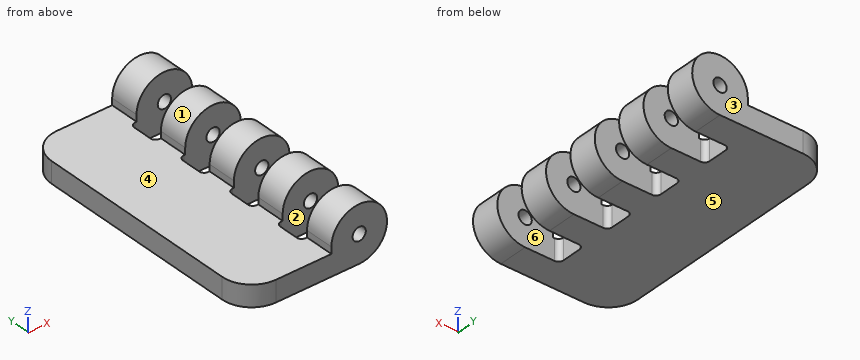
```python
from build123d import *

# Parameters (mm, degrees)
BOSS_EXTRUDE1_START = 31.75
SKETCH3_R           = 1.5875
BOSS_EXTRUDE1_DEPTH = 63.5
FILLET1_R           = 7.055555556
SKETCH5_W           = 16.383
SKETCH5_H           = 7.055555556
CUT_EXTRUDE1_DEPTH  = 43.200038063
LPATTERN1_COUNT     = 5
LPATTERN1_PITCH     = 14.111111111
FILLET2_R           = 1.175925926
SKETCH6_W           = 16.383
SKETCH6_H           = 7.055555555
CUT_EXTRUDE2_DEPTH  = 43.200038063
LPATTERN2_COUNT     = 4
LPATTERN2_PITCH     = 14.111111111
FILLET3_R           = 1.175925926
FILLET4_R           = 0.391975309
BOSS_EXTRUDE3_START = 31.75
SKETCH7_R           = 1.5875
BOSS_EXTRUDE3_DEPTH = 63.5


with BuildPart() as part:
    # Sketch3 → Boss-Extrude1 (new body)
    with BuildSketch(Plane(origin=(0, 0, 0), x_dir=(1, 0, 0), z_dir=(0, 1, 0)).offset(BOSS_EXTRUDE1_START)):
        with BuildLine():
            Line((26.9875, 6.6675), (26.9875, 1.5875))
            Line((26.9875, 1.5875), (6.6675, 1.5875))
            Line((6.6675, 1.5875), (6.6675, 0))
            ThreePointArc((6.6675, 0), (-4.714634464, -4.714634464), (0, 6.6675))
            Line((0, 6.6675), (26.9875, 6.6675))
        make_face()
        with Locations(Location((0, 0, 0), (0, 0, 270))):
            Circle(SKETCH3_R, mode=Mode.SUBTRACT)
    extrude(amount=-BOSS_EXTRUDE1_DEPTH)

    # Fillet1
    fillet1_edges = [part.edges().sort_by_distance(p)[0] for p in [
        (26.9875, -31.75, -4.1275),
        (26.9875, 31.75, -4.1275),
    ]]
    fillet(fillet1_edges, radius=FILLET1_R)


with BuildPart() as body_2:
    # Mirror1: mirrored copy
    add(part.part.mirror(Plane(origin=(0, 0, 0), x_dir=(0, 0, 1), z_dir=(1, 0, 0))))

    # Sketch6 → Cut-Extrude2 (cut, symmetric)
    with BuildSketch(Plane.XY):
        with Locations((0, 21.166666666)):
            Rectangle(SKETCH6_W, SKETCH6_H)
    cut_extrude2 = extrude(amount=CUT_EXTRUDE2_DEPTH, both=True, mode=Mode.SUBTRACT)

    # LPattern2: Cut-Extrude2 ×4
    with Locations(*[(0, -i * LPATTERN2_PITCH, 0) for i in range(1, LPATTERN2_COUNT)]):
        add(cut_extrude2, mode=Mode.SUBTRACT)

    # Fillet3
    fillet3_edges = [body_2.edges().sort_by_distance(p)[0] for p in [
        (-8.1915, 10.583333333, -4.1275),
        (-8.1915, 3.527777778, -4.1275),
        (-8.1915, -3.527777778, -4.1275),
        (-8.1915, -10.583333333, -4.1275),
        (-8.1915, -17.638888889, -4.1275),
        (-8.1915, -24.694444444, -4.1275),
        (-8.1915, 24.694444444, -4.1275),
        (-8.1915, 17.638888889, -4.1275),
    ]]
    fillet(fillet3_edges, radius=FILLET3_R)


with BuildPart() as part_1:
    add(part.part)

    # Sketch5 → Cut-Extrude1 (cut, symmetric)
    with BuildSketch(Plane.XY):
        with Locations((0, 28.222222222)):
            Rectangle(SKETCH5_W, SKETCH5_H)
    cut_extrude1 = extrude(amount=CUT_EXTRUDE1_DEPTH, both=True, mode=Mode.SUBTRACT)

    # LPattern1: Cut-Extrude1 ×5
    with Locations(*[(0, -i * LPATTERN1_PITCH, 0) for i in range(1, LPATTERN1_COUNT)]):
        add(cut_extrude1, mode=Mode.SUBTRACT)

    # Fillet2
    fillet2_edges = [part_1.edges().sort_by_distance(p)[0] for p in [
        (8.1915, -3.527777778, -4.1275),
        (8.1915, 3.527777778, -4.1275),
        (8.1915, -17.638888889, -4.1275),
        (8.1915, -10.583333333, -4.1275),
        (8.1915, -24.694444444, -4.1275),
        (8.1915, 24.694444444, -4.1275),
        (8.1915, 10.583333333, -4.1275),
        (8.1915, 17.638888889, -4.1275),
    ]]
    fillet(fillet2_edges, radius=FILLET2_R)

    # Fillet4
    fillet4_edges = [part_1.edges().sort_by_distance(p)[0] for p in [
        (8.1915, -31.75, -4.1275),
        (8.1915, 31.75, -4.1275),
    ]]
    fillet(fillet4_edges, radius=FILLET4_R)


with BuildPart() as body_3:
    # Sketch7 → Boss-Extrude3 (new body)
    with BuildSketch(Plane(origin=(0, 0, 0), x_dir=(1, 0, 0), z_dir=(0, 1, 0)).offset(BOSS_EXTRUDE3_START)):
        with Locations(Location((0, 0, 0), (0, 0, 270))):
            Circle(SKETCH7_R)
    extrude(amount=-BOSS_EXTRUDE3_DEPTH)


solid = body_2.part
```
Source: CAD feature listing. Evaluate the final solid. Frame: model axes, mm. Face numbers are marked on the shaded views. A direction names the side the tool comes from. Give positions to 0.01 mm unless a question says otherwise; leave off trailing zeros. Order: outer loops, then holes, each group sorted by start corner. A loop starts at its lowest first (then second) coordinate and runs counter-clockwise, first axis right, second up.
(1) Section query C-C (x = 3). Return the cut outline in (y, z).
(2) Access query for the marked faces 4, 5 and 6. Directions: +Z, -Z, +X, -X, +Y, -Y. A direction counts if a zero-diameter tool reaches every point of the face in a straight line with its end or side. Return the directions, or none.
(3) Section query D-D (y = 7.5). Return the cut outline in (x, z), plus the area to 3 significant figures.
(4) Pull-direction query (Y, two-part tool) for the marked faces 1, 2 and 3; classes: +Y half, -Y half, draft (parallel to the pull), parting line (faces both ways), or undercut.
(5) Section query A-A (z = 5.5). Return the cut outline in (x, y), plus the area to 3 significant figures.
(6) Section query B-B (y = 16). Return the cut outline in (x, z) (1 decimal).
(7) Material intervals for line 1 along Y through (x, z) = (1, 2.5); line 2 along X through (y, z) = (-1.75, 0); line 3 along Y through (x, z) = (-8, -2.75), sorted ascending.
(8) Contact query for flat-ended pins moving along their axis: P1, Ø1, axis at y = -21.5, z = -3.5, coming from the +X side; P2, Ø0.8, axis at y = -27, z = -0.5, coming from the -X side; P3, Ø2, axis at y = 1.5, z = -1.5, coming from the +X side. Output: stop coordinate, or through.
Outcome:
1. outline: (-31.75, -5.95) - (-24.69, -5.95) - (-24.69, 5.95) - (-31.75, 5.95) - close; (-17.64, -5.95) - (-10.58, -5.95) - (-10.58, 5.95) - (-17.64, 5.95) - close; (-3.53, -5.95) - (3.53, -5.95) - (3.53, 5.95) - (-3.53, 5.95) - close; (10.58, -5.95) - (17.64, -5.95) - (17.64, 5.95) - (10.58, 5.95) - close; (24.69, -5.95) - (31.75, -5.95) - (31.75, 5.95) - (24.69, 5.95) - close
2. face 4: +Z, -X, +Y, -Y
2. face 5: -Z, +X, -X, +Y, -Y
2. face 6: +Z, -Z, +X
3. outline: (-26.99, -6.67) - (-8.19, -6.67) - (-8.19, -1.59) - (-26.99, -1.59) - close
3. area: 95.5 mm2
4. face 1: draft
4. face 2: undercut
4. face 3: +Y half
5. outline: (-3.77, -31.75) - (3.77, -31.75) - (3.77, -24.69) - (-3.77, -24.69) - close; (-3.77, -17.64) - (3.77, -17.64) - (3.77, -10.58) - (-3.77, -10.58) - close; (-3.77, -3.53) - (3.77, -3.53) - (3.77, 3.53) - (-3.77, 3.53) - close; (-3.77, 10.58) - (3.77, 10.58) - (3.77, 17.64) - (-3.77, 17.64) - close; (-3.77, 24.69) - (3.77, 24.69) - (3.77, 31.75) - (-3.77, 31.75) - close
5. area: 266 mm2
6. outline: (-27, -6.7) - (0, -6.7) arc R6.7 ccw (long way) to (-6.7, 0) - (-6.7, -1.6) - (-27, -1.6) - close; hole circle Ø3.2 at (0, 0)
7. line 1: y = -31.75 to -24.69, -17.64 to -10.58, -3.53 to 3.53, 10.58 to 17.64, 24.69 to 31.75
7. line 2: x = -6.67 to -1.59, 1.59 to 6.67
7. line 3: y = -31.75 to -24.16, -18.17 to -10.05, -4.06 to 4.06, 10.05 to 18.17, 24.16 to 31.75
8. P1: stops at x = -8.19
8. P2: stops at x = -6.67
8. P3: stops at x = 6.65
